Can you work these out from the model? Positions are in its coordinate system, mm. Face numbers are marked on the shaded views. Coordinates: 2 decimals unless noted, no trailing zeros. Order: outer loops, then holes, each group sorted by start corner. A loop starts at its lowest first (then second) coordinate and runs counter-clockwise, first axis right, second up. Notation, with made-up numbers: (70, 31.5) -> (97, 31.5) arc R10 ccw to (97, 48.5) -> close; hole circle Ø8 at (69.25, -4). An arc over 180 degrees is marked (long way). Use a Markdown table: item, result. Add a question column.
1. Suppose I cut it at B-B, the plane x = 2.25. List the corners of the cut face in (y, z) for me, then the cut area to 3 significant figures.
2. We'd pull the mould along Y, two halves only. Please class the marked faces 1, 2, 3 and 4: pulls with the +Y half, pulls with the -Y half, needs draft (parallel to the pull), parting line crosses it, or undercut.
3. For pin 1 Ø1.5 at (x, y) = (1, 3) entering from +Z, with a flat end and sliding along its axis, tell me the tip position at first contact or that it passes through.
4. Suppose I cut it at C-C, the plane z = 70.5. List the corners of the cut face in (x, y) for me, then the cut area to 3 significant figures.
5. Suppose I cut it at A-A, the plane y = 0. List the corners of the cut face in (x, z) for me, then the cut area to 3 significant figures.
6. If I drill on line 1 along Y through (x, z) = (0, 34); line 2 along Y through (x, z) = (3, 69); line 3 along X through (y, z) = (0.5, 75), over which ranges is the centre line in solid material (lowest first)? Write a range as from..to.
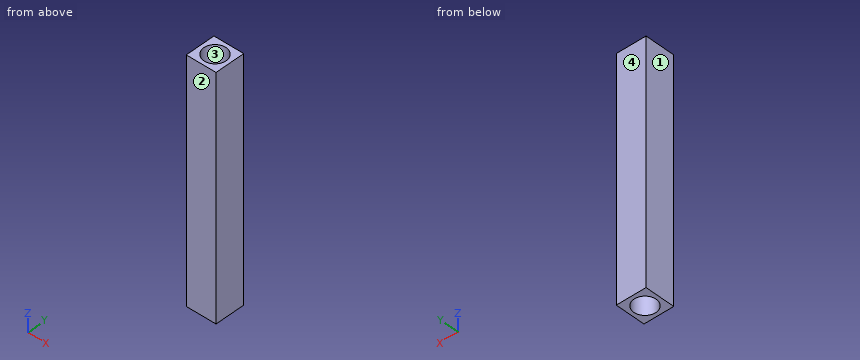
```python
from build123d import *

# Parameters (mm, degrees)
F0_W      = 10
F0_H      = 10
F0_R      = 3.75
F1_DEPTH  = 70
F1_FACE_W = 10
F1_FACE_H = 10
F1_FACE_R = 3.75
F2_DEPTH  = 10


with BuildPart() as f1:
    # F0 (on Top) → F1 (new body)
    with BuildSketch(Plane.XY):
        Rectangle(F0_W, F0_H)
        Circle(F0_R, mode=Mode.SUBTRACT)
    extrude(amount=F1_DEPTH)

    # F1_face (on face) → F2 (join)
    with BuildSketch(Plane.XY.offset(70)):
        Rectangle(F1_FACE_W, F1_FACE_H)
        Circle(F1_FACE_R, mode=Mode.SUBTRACT)
    extrude(amount=F2_DEPTH)


solid = f1.part
```
Worked out:
| question | item | result |
|---|---|---|
| 1 | outline | (-5, 0) -> (-3, 0) -> (-3, 80) -> (-5, 80) -> close; (3, 0) -> (5, 0) -> (5, 80) -> (3, 80) -> close |
| 1 | area | 320 mm² |
| 2 | face 1 | needs draft |
| 2 | face 2 | pulls with the -Y half |
| 2 | face 3 | undercut |
| 2 | face 4 | pulls with the +Y half |
| 3 | pin 1 | stops at z = 80 |
| 4 | outline | (-5, -5) -> (5, -5) -> (5, 5) -> (-5, 5) -> close; hole circle Ø7.5 at (0, 0) |
| 4 | area | 55.8 mm² |
| 5 | outline | (-5, 0) -> (-3.75, 0) -> (-3.75, 80) -> (-5, 80) -> close; (3.75, 0) -> (5, 0) -> (5, 80) -> (3.75, 80) -> close |
| 5 | area | 200 mm² |
| 6 | line 1 | y = -5..-3.75, 3.75..5 |
| 6 | line 2 | y = -5..-2.25, 2.25..5 |
| 6 | line 3 | x = -5..-3.72, 3.72..5 |
